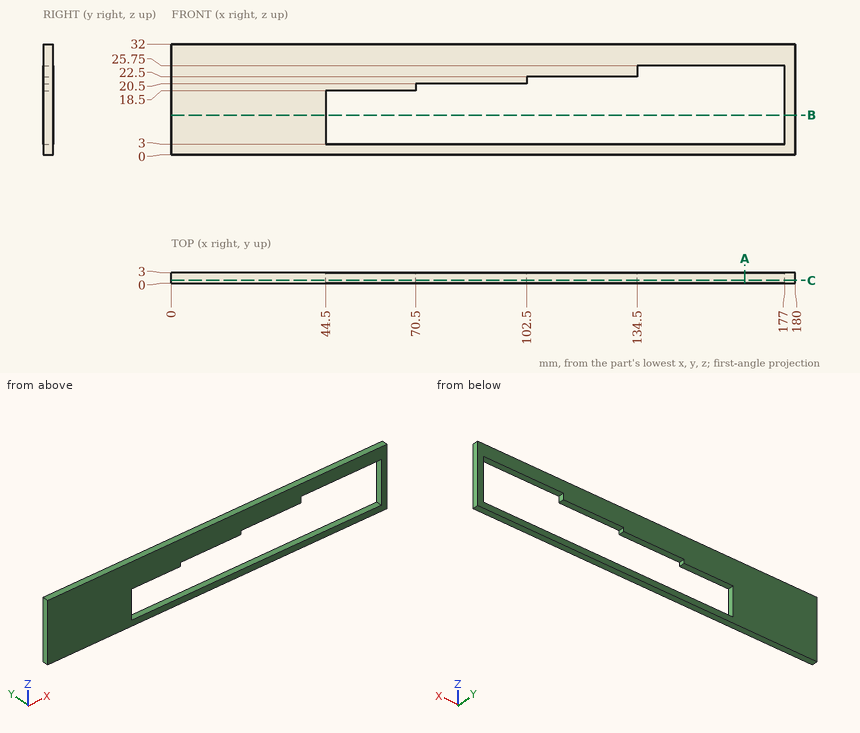
Geometry check sheet. Reference: drawing and pictorial views, mm from the part's lowest x, y, z. Give positions to 0.01 mm unless a question says otherwise; leave off trailing zeros. Order: outer loops, then holes, each group sorted by start corner. A loop starts at its lowest first (then second) coordinate and runs counter-clockwise, first axis right, second up. Notation, with made-up numbers: M 38.25,23 L 88.25,23 A28 cw 88.25,42 Z; hole C 28.5,49 d9. An arc over 180 degrees is marked long. Use one line per item in the form item = value. Start each with the question number.
Q1. Section check C-C (y = 0.8). Enter the section's corners in (x, z), then the cut area to 3 significant figures.
Q2. Section check A-A (x = 165.5). Enter the section's corners in (y, z).
Q3. Scan lines: line 1 along Z through (x, y) = (118, 0.8); line 2 along X through (y, z) = (2.15, 7.5); line 3 along Z through (x, y) = (155, 2.65). Record each from-to range of solid material in increasing order. Write a range as [from, to].
Q4. Section check B-B (z = 11.5). Enter the section's corners in (x, y), then the cut area to 4 significant figures.
Evaluation:
q1.outline = M 0,0 L 180,0 L 180,32 L 0,32 Z; hole M 44.5,3 L 177,3 L 177,25.75 L 134.5,25.75 L 134.5,22.5 L 102.5,22.5 L 102.5,20.5 L 70.5,20.5 L 70.5,18.5 L 44.5,18.5 Z
q1.area = 3,210 mm2
q2.outline = M 0,0 L 3,0 L 3,3 L 0,3 Z; M 0,25.75 L 3,25.75 L 3,32 L 0,32 Z
q3.line_1 = [0, 3], [22.5, 32]
q3.line_2 = [0, 44.5], [177, 180]
q3.line_3 = [0, 3], [25.75, 32]
q4.outline = M 0,0 L 44.5,0 L 44.5,3 L 0,3 Z; M 177,0 L 180,0 L 180,3 L 177,3 Z
q4.area = 142.5 mm2
